```python
from build123d import *

# Parameters (mm, degrees)
SKETCH1_R           = 70
BOSS_EXTRUDE1_DEPTH = 40
SKETCH3_W           = 6.5
SKETCH3_H           = 32.4
SKETCH5_W           = 9.259396931
SKETCH5_H           = 5.5
SKETCH6_W           = 156.018137672
SKETCH6_H           = 46.428345924
CUT_EXTRUDE1_DEPTH  = 81


with BuildPart() as part:
    # Sketch1 → Boss-Extrude1 (new body, symmetric)
    with BuildSketch(Plane.XY):
        Circle(SKETCH1_R)
    extrude(amount=BOSS_EXTRUDE1_DEPTH, both=True)

    # Sketch2 → Cut-Revolve1 (revolve, cut)
    with BuildSketch(Plane(origin=(0, 0, 0), x_dir=(1, 0, 0), z_dir=(0, 1, 0))):
        Polygon((-69, 40), (-69, 35), (-67, 35), (-67, 28.7), (-60, 28.7), (-60, 3.7), (-67, 3.7), (-67, -2.6), (-69, -2.6), (-69, -44.705491592), (-73.643536697, -44.705491592), (-73.643536697, 40), align=None)
    revolve(axis=Axis((0, 0, 0), (0, 0, -1)), mode=Mode.SUBTRACT)

    # Sketch3 → Cut-Revolve2 (revolve, cut)
    with BuildSketch(Plane(origin=(0, 0, 0), x_dir=(1, 0, 0), z_dir=(0, 1, 0))):
        with Locations((-65.75, -23.8)):
            Rectangle(SKETCH3_W, SKETCH3_H)
    revolve(axis=Axis((0, 0, 0), (0, 0, 1)), mode=Mode.SUBTRACT)

    # Sketch4 → Cut-Revolve3 (revolve, cut)
    with BuildSketch(Plane(origin=(0, 0, 0), x_dir=(1, 0, 0), z_dir=(0, 1, 0))):
        Polygon((0, 42.623044552), (-37.5, 42.623044552), (-37.5, 20), (-33, 20), (-33, -40), (0, -40), align=None)
    revolve(axis=Axis((0, 0, 0), (0, 0, -1)), mode=Mode.SUBTRACT)

    # Sketch5 → Cut-Revolve4 (revolve, cut)
    with BuildSketch(Plane(origin=(0, 0, 0), x_dir=(1, 0, 0), z_dir=(0, 1, 0))):
        with Locations((-37.620301535, 32.25)):
            Rectangle(SKETCH5_W, SKETCH5_H)
    revolve(axis=Axis((0, 0, 0), (0, 0, -1)), mode=Mode.SUBTRACT)

    # Sketch6 → Cut-Extrude1 (cut, symmetric)
    with BuildSketch(Plane(origin=(0, 0, 0), x_dir=(1, 0, 0), z_dir=(0, 1, 0))):
        with Locations((-2.837222121, 26.914172962)):
            Rectangle(SKETCH6_W, SKETCH6_H)
    extrude(amount=CUT_EXTRUDE1_DEPTH, both=True, mode=Mode.SUBTRACT)


solid = part.part
```
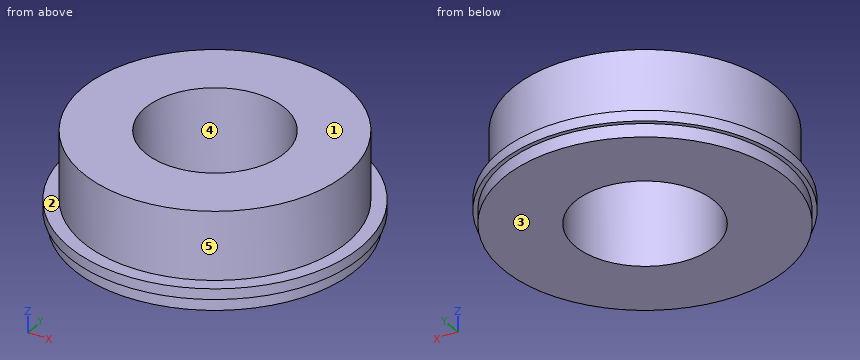
The listing builds one solid part. Answer for the finished solid, in the listing's coordinates (mm). Face numbers are marked on the shaded views. A direction names the side the tool comes from. Give positions to 0.01 mm unless a question says otherwise; leave off trailing zeros. Order: outer loops, then holes, each group sorted by start corner. A loop starts at its lowest first (then second) coordinate and runs counter-clockwise, first axis right, second up. Notation, with made-up numbers: (66.25, -3.5) -> (104.25, -3.5) arc R14 cw to (104.25, 1.5) -> close; hole circle Ø2 at (87.25, 23). An arc over 180 degrees is marked (long way). Answer as a JSON object with one key per item and string values. Group by question number.
Item 1: Determine the mould class of the marked faces 3, 4 and 5 for opening direction X: pulls with the +X half, pulls with the -X half, needs draft (parallel to the pull), parting line crosses it, or undercut.
Item 2: The part is cut by section C-C on x = -36. Write down the section's boundary in (y, z).
Item 3: Flat-ended cylindrical pins translate along their axes: pin 1 (2 mm diameter, centred on y = 44.5, z = 18.5, fed in from +X); pin 2 (10 mm diameter, centred on x = 44.5, z = 6.5, fed in from +Y); pin 3 (8 mm diameter, centred on y = -42, z = 28.5, fed in from -X). Find the tip coordinate at first contact, or state that the pin passes through.
Item 4: The part is cut by section D-D on y = -54.5. Write down the section's boundary in (x, z), and give its area (3 significant figures).
Item 5: The part is cut by section A-A on y = 0. Write down the section's boundary in (x, z).
Item 6: Consider L1, parallel to X at y = 0, z = 12; L2, parallel to Y at x = 0, z = 7. Determine where each line is inside the solid, lowest interval first. Write a range as from..to.
Item 7: A tool of negligible diameter and unlimited length cuts with its end or side. For the marked faces 1 and 2, from which of +Z, -Z, +X, -X, +Y, -Y can it reach the whole face along a straight path? Write none if from no direction.
Result set:
{
 "1": {"face 3": "needs draft", "face 4": "undercut", "face 5": "parting line crosses it"},
 "2": {"outline": "(-58.86, 2.6) -> (-56.51, 2.6) -> (-56.51, -3.7) -> (56.51, -3.7) -> (56.51, 2.6) -> (58.86, 2.6) -> (58.86, 7.6) -> (51.09, 7.6) -> (51.09, 40) -> (-51.09, 40) -> (-51.09, 7.6) -> (-58.86, 7.6) -> close"},
 "3": {"pin 1": "x = 44.88", "pin 2": "y = 56.58", "pin 3": "x = -49.62"},
 "4": {"outline": "(-42.32, 2.6) -> (-38.97, 2.6) -> (-38.97, -3.7) -> (38.97, -3.7) -> (38.97, 2.6) -> (42.32, 2.6) -> (42.32, 7.6) -> (30.59, 7.6) -> (30.59, 40) -> (-30.59, 40) -> (-30.59, 7.6) -> (-42.32, 7.6) -> close", "area": "2,900 mm²"},
 "5": {"outline": "(-69, 2.6) -> (-67, 2.6) -> (-67, -3.7) -> (-33, -3.7) -> (-33, 40) -> (-62.5, 40) -> (-62.5, 7.6) -> (-69, 7.6) -> close; (33, -3.7) -> (67, -3.7) -> (67, 2.6) -> (69, 2.6) -> (69, 7.6) -> (62.5, 7.6) -> (62.5, 40) -> (33, 40) -> close"},
 "6": {"L1": "-62.5..-33, 33..62.5", "L2": "-69..-33, 33..69"},
 "7": {"face 1": "+Z, +X, -X, +Y, -Y", "face 2": "+Z"}
}
